Part print with two shaded views. Sizes in mm from the minimum x, y, z corner. A direction names the side the tool comes from. Round coordinates to 2 decimals unless told otherwise and drop trailing zeros. Answer as CSV lines item,"result". Start each with the question number.
Item 1: Which spindle directions (+Z, -Z, +X, -X, +Y, -Y) get a long thin tool onto all of the face, cutting with end or side? Do the marked faces 4, 5 and 6. Say none if no direction does.
Item 2: Mould opens along Y. For the marked faces 1, 2 and 3 say: pulls with the +Y half, pulls with the -Y half, needs draft (parallel to the pull), parting line crosses it, or undercut.
Item 3: Band-saw the part on A-A (z = 73). Count the separate pieces of the cut face and the enclosed holes in it, and give its area (3 significant figures).
Item 4: Wall check: line 1 (X direction, y = 19.25, z = 40); line 2 (Z direction, x = 40, y = 8); line 3 (Z direction, x = 29, y = 24.75) (1 decimal). Give the ranges that are in metal, low to high.
Item 5: Drop flat-ended pins along their axis: pin 1 Ø3 at (y, z) = (15.5, 53) entering from -X (1 decimal); pin 2 Ø1.5 at (x, z) = (61.5, 61.5) entering from -Y; pin 3 Ø6 at (y, z) = (23, 18) entering from +X; pin 4 Ø3 at (y, z) = (3.5, 59.5) entering from +X. Give the stop position or say it passes through.
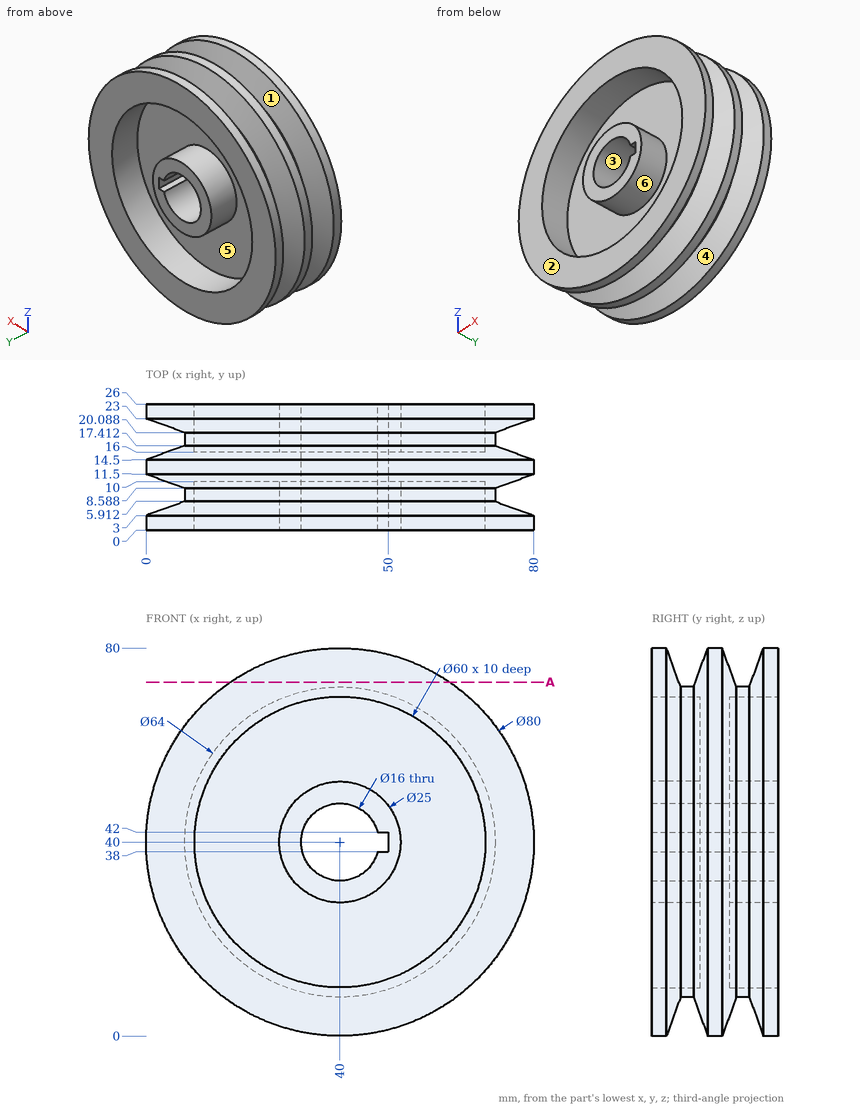
Answer block:
1,face 4,"none"
1,face 5,"+Y"
1,face 6,"-Y"
2,face 1,"undercut"
2,face 2,"pulls with the -Y half"
2,face 3,"needs draft"
3,separate pieces,"3"
3,enclosed holes,"0"
3,area,"708 mm^2"
4,line 1,"x = 8 to 10, 27.5 to 32, 50 to 52.5, 70 to 72"
4,line 2,"z = 8 to 10, 27.5 to 32, 48 to 52.5, 70 to 72"
4,line 3,"z = 1.5 to 12.1, 34.1 to 45.9, 67.9 to 78.5"
5,pin 1,"stops at x = 1.8"
5,pin 2,"stops at y = 0"
5,pin 3,"stops at x = 75.2"
5,pin 4,"stops at x = 75.68"
